```python
from build123d import *

# Parameters (mm, degrees)
SKETCH1_R           = 33.14
BOSS_EXTRUDE7_DEPTH = 40
SKETCH4_R           = 17.5
CUT_EXTRUDE1_DEPTH  = 5
BOSS_EXTRUDE9_DEPTH = 8
SKETCH7_R           = 6
CUT_EXTRUDE2_DEPTH  = 178.288271755


# Read off the part's stored shape, not the designer's step: Boss-Extrude8
with BuildPart() as part:
    # Sketch1 → Boss-Extrude7 (new body)
    with BuildSketch(Plane(origin=(0, 0, 0), x_dir=(1, 0, 0), z_dir=(0, 1, 0))):
        with Locations(Location((0, 0, 0), (0, 0, 270))):
            Circle(SKETCH1_R)
    extrude(amount=BOSS_EXTRUDE7_DEPTH)

    # Sketch2 → Cut-Revolve1 (revolve, cut)
    with BuildSketch(Plane.XY):
        with BuildLine():
            Line((0, 33.14), (0, 0))
            Line((0, 0), (33.14, 0))
            ThreePointArc((33.14, 0), (23.433518729, 23.433518729), (0, 33.14))
        make_face()
    revolve(axis=Axis((0, 33.14, 0), (0, -1, 0)), mode=Mode.SUBTRACT)

    # Sketch4 → Cut-Extrude1 (cut)
    with BuildSketch(Plane(origin=(0, 40, 0), x_dir=(1, 0, 0), z_dir=(0, 1, 0))):
        with Locations(Location((0, 0, 0), (0, 0, 270))):
            Circle(SKETCH4_R)
    extrude(amount=-CUT_EXTRUDE1_DEPTH, mode=Mode.SUBTRACT)

    # Boss-Extrude8 outline → Boss-Extrude8 (revolve)
    with BuildSketch(Plane.XY):
        Polygon((17.5, 35), (17.5, 50), (10.507318806, 150), (0, 150), (0, 35), align=None)
    revolve(axis=Axis((0, 0, 0), (0, 1, 0)))

    # Sketch6 → Boss-Extrude9 (add)
    with BuildSketch(Plane(origin=(0, 150, 0), x_dir=(1, 0, 0), z_dir=(0, 1, 0))):
        Polygon((0, 7.07), (-7.072135463, 0), (0, -7.07), (7.072135463, 0), align=None)
    extrude(amount=BOSS_EXTRUDE9_DEPTH)

    # Sketch7 → Cut-Extrude2 (cut, through all)
    with BuildSketch(Plane(origin=(-0.293937447, 0, 39.998930323), x_dir=(0.9999729998922554, 0, 0.007348434287890893), z_dir=(-0.007348434287890893, -1.1102230246251565e-15, 0.9999729998922554))):
        with Locations(Location((0, 128, 0), (0, 0, 270.874748169))):
            Circle(SKETCH7_R)
    extrude(amount=-CUT_EXTRUDE2_DEPTH, mode=Mode.SUBTRACT)


solid = part.part
```
The model under review builds one solid part; all positions refer to its coordinate system, in mm. A direction names the side the tool comes from. Round coordinates to 2 decimals unless told otherwise and drop trailing zeros. Order: outer loops, then holes, each group sorted by start corner. A loop starts at its lowest first (then second) coordinate and runs counter-clockwise, first axis right, second up. Notation, with made-up numbers: M -27.5,82 L 2.5,82 A15 cw 2.5,110 Z; hole C 75.25,79.5 d5. An arc over 180 degrees is marked long. Use a Markdown table: item, result.
1) Consider section A-A (y = 11). Write out the cut boundary in (x, z).
Report:
| item | result |
|---|---|
| outline | C 0,0 d66.28; hole C 0,0 d62.52 |
2) Consider section C-C (x = -19). Write out the cut boundary in (y, z).
Report:
| item | result |
|---|---|
| outline | M 0,-27.15 L 40,-27.15 L 40,27.15 L 0,27.15 A27.15 cw Z |
3) Consider section B-B (y = 48). Write out the cut boundary in (x, z), then the cut area to 3 significant figures.
Report:
| item | result |
|---|---|
| outline | C 0,0 d35 |
| area | 962 mm^2 |
4) Consider section D-D (z = 23). Write out the cut boundary in (x, y), then the cut area to 3 significant figures.
Report:
| item | result |
|---|---|
| outline | M -23.86,0 A23.86 cw 23.86,0 L 23.86,40 L -23.86,40 Z |
| area | 1,010 mm^2 |
5) Insertion check: pin 1 (1 mm diameter, centred on y = 132, z = -6, fed in from +X); pin 2 (6 mm diameter, centred on y = 130.5, z = -2.5, fed in from -X); pin 3 (8 mm diameter, centred on y = 64, z = -6.5, fed in from +X). Each pin has a flat end and moves straight along its axis. Give the tip position at first contact, or say it passes through.
Report:
| item | result |
|---|---|
| pin 1 | x = 10.4 |
| pin 2 | x = -12.02 |
| pin 3 | x = 16.39 |
6) Tool access review of faces 5 (the face through (-14, 40, 14)), 6 (the face through (-3.49, 153.94, -3.58)), 7 (the face through (3.586, 153.944, -3.486)): name each direction out of +Z, -Z, +X, -X, +Y, -Y from which nothing blocks a thin tool from reaching the whole face with its end or side.
Report:
| item | result |
|---|---|
| face 5 | +Y |
| face 6 | -Z, -X, +Y |
| face 7 | -Z, +X, +Y |
7) Wall thickness on line 1 along Y through (x, z) = (4.5, 9); line 2 along Y through (x, z) = (-4, 26); line 3 along Z through (x, y) = (-10, 102): over which ranges is each line inside the solid? List them lowest first. Write a range as [from, to].
Report:
| item | result |
|---|---|
| line 1 | [31.58, 124.11], [131.89, 150] |
| line 2 | [20.16, 40] |
| line 3 | [-9.6, 9.6] |
8) Draft analysis for pull direction X (two halves, no side actions). For faces 1 (the face through (-3.586, 153.944, 3.486)), 2 (the face through (16.69, 45.07, -5.26)), 3 (the face through (3.49, 153.94, 3.58)), 4 (the face through (1.888, 122.305, 0.188)), state which applies: released by +X, released by -X, zero draft, split by the parting line, or undercut.
Report:
| item | result |
|---|---|
| face 1 | released by -X |
| face 2 | split by the parting line |
| face 3 | released by +X |
| face 4 | undercut |
